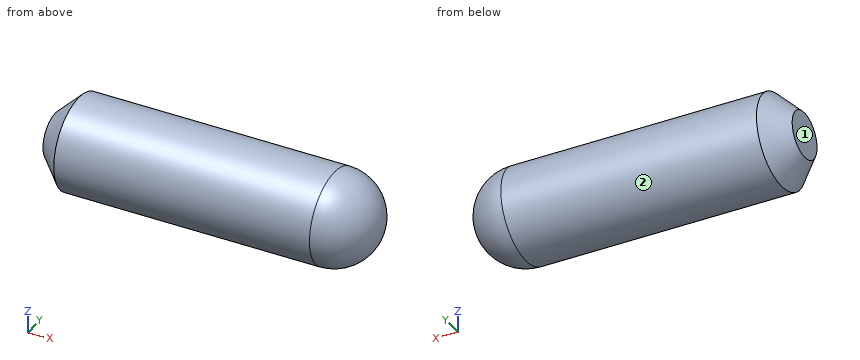
```python
from build123d import *

# Parameters (mm, degrees)
SKETCH1_W     = 14
SKETCH1_H     = 2
CHAMFER1_SIZE = 1
FILLET1_R     = 2


with BuildPart() as part:
    # Sketch1 → Revolve1 (revolve)
    with BuildSketch(Plane.XY):
        with Locations((7, 1)):
            Rectangle(SKETCH1_W, SKETCH1_H)
    revolve(axis=Axis((-4.801500481, 0, 0), (1, 0, 0)))

    # Chamfer1
    chamfer1_edges = [part.edges().sort_by_distance(p)[0] for p in [
        (0, -2, 0),
    ]]
    chamfer(chamfer1_edges, length=CHAMFER1_SIZE)

    # Fillet1
    fillet1_edges = [part.edges().sort_by_distance(p)[0] for p in [
        (14, -2, 0),
    ]]
    fillet(fillet1_edges, radius=FILLET1_R)


solid = part.part
```
Source: CAD feature listing. Evaluate the final solid. Frame: model axes, mm. Face numbers are marked on the shaded views. Round coordinates to 2 decimals unless told otherwise and drop trailing zeros. Loops run counter-clockwise (first coordinate to the right, second up) from the corner with the lowest first, then second, coordinate; pieces in that order, holes last. Notation, with made-up numbers: M 3.25,19.25 L 56.25,19.25 A23 ccw 56.25,34.25 Z; hole C 85.25,-30 d6. An arc over 180 degrees is marked long. Use a Markdown table: item, result. Add a question column.
1. Contact query for flat-ended pins moving along their axis: pin 1 (1 mm diameter, centred on x = 7.5, z = -1, fed in from +Y); pin 2 (1 mm diameter, centred on y = 0.5, z = 1.5, fed in from +X). Output: stop coordinate, or through.
2. Cut plane D-D, the plane x = 12.75. Output: boundary loops of the cut face in (y, z).
3. Cut plane C-C, the plane x = 2.5. Output: boundary loops of the cut face in (y, z).
4. Cut plane A-A, the plane y = 0. Output: boundary loops of the cut face in (x, z).
5. Ray query, line 1 along Y through (x, z) = (1.25, -0.1); line 2 along X through (y, z) = (0.1, -1.2); line 3 along Y through (x, z) = (13, 0.6). Return the intervals inside material, ascending. Write a range as [from, to].
6. Pull-direction query (Y, two-part tool) for the marked faces 1 and 2; classes: +Y half, -Y half, draft (parallel to the pull), parting line (faces both ways), or undercut.
Solution:
| question | item | result |
|---|---|---|
| 1 | pin 1 | stops at y = 1.94 |
| 1 | pin 2 | stops at x = 13.68 |
| 2 | outline | C 0,0 d3.71 |
| 3 | outline | C 0,0 d4 |
| 4 | outline | M 0,-1 L 1,-2 L 12,-2 A2 ccw 12,2 L 1,2 L 0,1 Z |
| 5 | line 1 | y = [-2, 2] |
| 5 | line 2 | x = [0.2, 13.6] |
| 5 | line 3 | y = [-1.62, 1.62] |
| 6 | face 1 | draft |
| 6 | face 2 | parting line |
